Geometry check sheet. Reference: the model listing, model coordinates, mm. Face numbers are marked on the shaded views. A direction names the side the tool comes from. Coordinates: 2 decimals unless noted, no trailing zeros. Loops run counter-clockwise (first coordinate to the right, second up) from the corner with the lowest first, then second, coordinate; pieces in that order, holes last. Notation, with made-up numbers: (9.25, -3.5) - (13.25, -3.5) arc R35 ccw to (13.25, 30.5) - close; hole circle Ø10 at (23, 45). An arc over 180 degrees is marked (long way). One line per item, written item: value.
from build123d import *

# Parameters (mm, degrees)
CROQUIS1_W              = 30
CROQUIS1_H              = 43
CROQUIS1_R              = 1.5
SALIENTE_EXTRUIR1_DEPTH = 3
CROQUIS2_W              = 60
CROQUIS2_H              = 70
CROQUIS2_R              = 1.5
SALIENTE_EXTRUIR2_DEPTH = 3


with BuildPart() as part:
    # Croquis1 → Saliente-Extruir1 (new body)
    with BuildSketch(Plane.XY):
        with Locations((-25.378630764, -5.032160817)):
            Rectangle(CROQUIS1_W, CROQUIS1_H)
        with Locations((-34.878630764, 11.467839183)):
            Circle(CROQUIS1_R, mode=Mode.SUBTRACT)
        with Locations((-34.878630764, -20.532160817)):
            Circle(CROQUIS1_R, mode=Mode.SUBTRACT)
    extrude(amount=SALIENTE_EXTRUIR1_DEPTH)

    # Croquis2 → Saliente-Extruir2 (add)
    with BuildSketch(Plane(origin=(-10.378630764, 0, 0), x_dir=(0, 0, -1), z_dir=(1, 0, 0))):
        with Locations((30, 8.467839183)):
            Rectangle(CROQUIS2_W, CROQUIS2_H)
        with Locations((57, 39.467839183)):
            Circle(CROQUIS2_R, mode=Mode.SUBTRACT)
        with Locations((14, 39.467839183)):
            Circle(CROQUIS2_R, mode=Mode.SUBTRACT)
        with Locations((14, -14.532160817)):
            Circle(CROQUIS2_R, mode=Mode.SUBTRACT)
        with Locations((57, -14.532160817)):
            Circle(CROQUIS2_R, mode=Mode.SUBTRACT)
    extrude(amount=-SALIENTE_EXTRUIR2_DEPTH)


solid = part.part
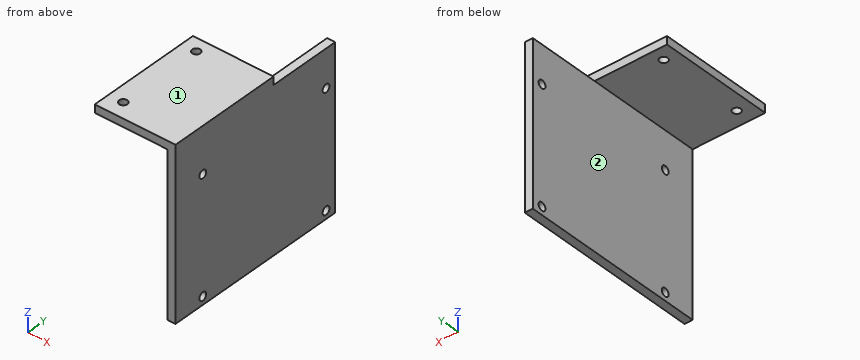
(1) Access from +Z, -Z, +X, -X, +Y, -Y to the whole of each face (thin tool, end or side, straight path). Record for the marked faces 1 and 2.
Reply:
face 1: +Z, +X, -X, +Y, -Y
face 2: -Z, -X, +Y, -Y
(2) Cross-section at B-B on y = -3. Record the cut outline in (x, z), and give its area (3 significant figures).
Reply:
outline: (-40.38, 0) - (-13.38, 0) - (-13.38, -60) - (-10.38, -60) - (-10.38, 3) - (-40.38, 3) - close
area: 270 mm2
(3) Cross-section at A-A on z = -57. Record the cut outline in (x, y).
Reply:
outline: (-13.38, -26.53) - (-10.38, -26.53) - (-10.38, -16.03) - (-13.38, -16.03) - close; (-13.38, -13.03) - (-10.38, -13.03) - (-10.38, 37.97) - (-13.38, 37.97) - close; (-13.38, 40.97) - (-10.38, 40.97) - (-10.38, 43.47) - (-13.38, 43.47) - close
(4) Cross-section at C-C on z = -7.5. Record the cut outline in (x, y).
Reply:
outline: (-13.38, -26.53) - (-10.38, -26.53) - (-10.38, 43.47) - (-13.38, 43.47) - close
(5) Go/stop test with flat-tipped pins: pin 1 Ø1.8 at (y, z) = (-14.53, -57) entering from -X; pin 2 Ø1.5 at (x, y) = (-12.5, 35) entering from +Z; pin 3 Ø1.5 at (y, z) = (14.5, -42.5) entering from -X; pin 4 Ø2.5 at (x, z) = (-19, 2) entering from +Y. Record where each tip stops, or that it passes through.
Reply:
pin 1: through
pin 2: z = 0
pin 3: x = -13.38
pin 4: y = 16.47
(6) Material ranges on probe 1 along Y at (x, z) = (-11.2, -57); probe 2 along Z at (x, y) = (-29.25, 16); probe 3 along X at (y, z) = (15, -31.5), recorded low to high. Write a range as from..to.
Reply:
probe 1: -26.53..-16.03, -13.03..37.97, 40.97..43.47
probe 2: 0..3
probe 3: -13.38..-10.38
(7) Cross-section at D-D on x = -15.25. Record the cut outline in (y, z), and give its area (3 significant figures).
Reply:
outline: (-26.53, 0) - (16.47, 0) - (16.47, 3) - (-26.53, 3) - close
area: 129 mm2
